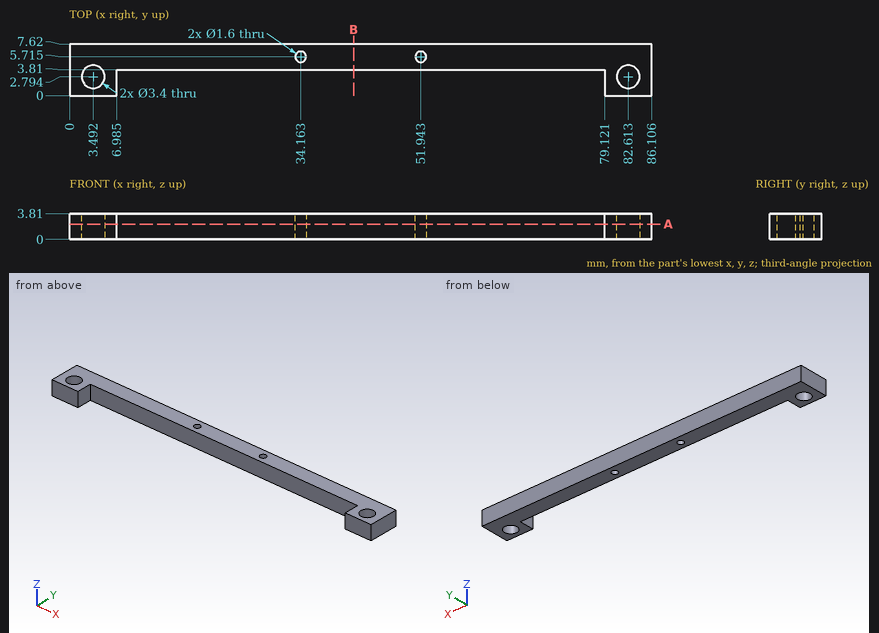
Here's the drawing with two shaded views (mm, measured from the low corner). I have some questions. Coordinates: 2 decimals unless noted, no trailing zeros. Loops run counter-clockwise (first coordinate to the right, second up) from the corner with the lowest first, then second, coordinate; pieces in that order, holes last. Notation, with made-up numbers: (17.25, 65.25) -> (73.25, 65.25) arc R28 ccw to (73.25, 86.25) -> close; hole circle Ø6 at (41.5, 16). An arc over 180 degrees is marked (long way). Use one line per item in the form item = value. Start each with the question number.
(1) Please list where these lines run through material, in increasing order: line 1 along X through (y, z) = (2.75, 0.75) (1 decimal); line 2 along X through (y, z) = (3.75, 2.1) (1 decimal); line 3 along X through (y, z) = (4.25, 2.2) (1 decimal).
(2) If we section it at A-A (z = 2.25): Please give me the cut outline in (x, y) (1 decimal).
(3) If we section it at B-B (x = 42): Please give me the cut outline in (y, z).
(4) Will this pin go through, and if not, where does the flat tip stop? pin 1 (1 mm diameter, centred on x = 15.5, z = 2.5, fed in from -Y).
Verdict:
q1.line_1 = 0 to 1.8, 5.2 to 7, 79.1 to 80.9, 84.3 to 86.1
q1.line_2 = 0 to 2.1, 4.9 to 7, 79.1 to 81.2, 84 to 86.1
q1.line_3 = 0 to 2.6, 4.4 to 81.7, 83.5 to 86.1
q2.outline = (0, 0) -> (7, 0) -> (7, 3.8) -> (79.1, 3.8) -> (79.1, 0) -> (86.1, 0) -> (86.1, 7.6) -> (0, 7.6) -> close; hole circle Ø3.4 at (3.5, 2.8); hole circle Ø1.6 at (34.2, 5.7); hole circle Ø1.6 at (51.9, 5.7); hole circle Ø3.4 at (82.6, 2.8)
q3.outline = (3.81, 0) -> (7.62, 0) -> (7.62, 3.81) -> (3.81, 3.81) -> close
q4.pin_1 = 3.81
